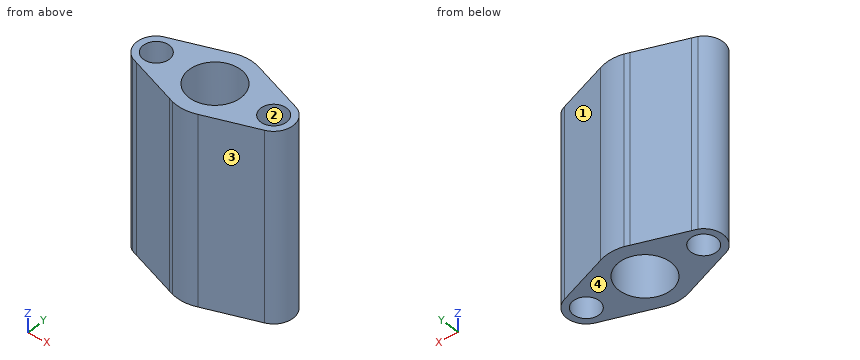
```python
from build123d import *

# Parameters (mm, degrees)
SKETCH5_R           = 10
SKETCH5_R_2         = 20
BOSS_EXTRUDE1_DEPTH = 147


with BuildPart() as part:
    # Sketch5 → Boss-Extrude1 (new body)
    with BuildSketch(Plane.XY):
        with BuildLine():
            Line((-95.000247062, 74.995110708), (-98.935518445, 73.594697295))
            ThreePointArc((-98.935518445, 73.594697295), (-106.987878642, 60.300702366), (-98.935518445, 47.006707437))
            Line((-98.935518445, 47.006707437), (-95.000247062, 45.606294025))
            Line((-95.000247062, 45.606294025), (-58.799859117, 32.723952789))
            Line((-58.799859117, 32.723952789), (-55.25219854, 31.46147532))
            ThreePointArc((-55.25219854, 31.46147532), (-45.821842976, 30.323371584), (-36.508384931, 32.190558084))
            Line((-36.508384931, 32.190558084), (3.010657963, 46.15804944))
            ThreePointArc((3.010657963, 46.15804944), (13.012121358, 60.300702366), (3.010657963, 74.443355293))
            Line((3.010657963, 74.443355293), (-36.508384931, 88.410846649))
            ThreePointArc((-36.508384931, 88.410846649), (-45.821842976, 90.278033149), (-55.25219854, 89.139929413))
            Line((-55.25219854, 89.139929413), (-58.799859117, 87.877451944))
            Line((-58.799859117, 87.877451944), (-95.000247062, 74.995110708))
        make_face()
        with Locations((-91.987878642, 60.300702366)):
            Circle(SKETCH5_R, mode=Mode.SUBTRACT)
        with Locations((-46.987878642, 60.300702366)):
            Circle(SKETCH5_R_2, mode=Mode.SUBTRACT)
        with Locations((-1.987878642, 60.300702366)):
            Circle(SKETCH5_R, mode=Mode.SUBTRACT)
    extrude(amount=-BOSS_EXTRUDE1_DEPTH)


solid = part.part
```
Part model, mm, in its own coordinate system. Face numbers are marked on the shaded views. Round coordinates to 2 decimals unless told otherwise and drop trailing zeros. Write each loop counter-clockwise with the first axis right and the second up, starting at its lowest first coordinate (ties: lowest second). Pieces come first, ordered by that corner, then holes. Notation, with made-up numbers: M -3,41 L 39,41 A16 cw 39,61 Z; hole C 84.25,74 d2. An arc over 180 degrees is marked long. One line per question, with ' | ' between items.
(1) Probe line 1 along X through (y, z) = (52, -51.5); line 2 along X through (y, z) = (64, -94.5); line 3 along Y through (x, z) = (-95.5, -21.5). List the from-to ranges inside material, lowest first.
Answer key:
line 1: x = -104.48 to -97.56, -86.41 to -65.18, -28.79 to -7.56, 3.59 to 10.51 | line 2: x = -106.52 to -101.28, -82.7 to -66.64, -27.33 to -11.28, 7.3 to 12.55 | line 3: y = 45.78 to 50.94, 69.66 to 74.82
(2) Saw through at B-B on z = -130. Write the cut outline in (x, y).
Answer key:
outline: M -98.94,47.01 L -55.25,31.46 A30 ccw -36.51,32.19 L 3.01,46.16 A15 ccw 3.01,74.44 L -36.51,88.41 A30 ccw -55.25,89.14 L -98.94,73.59 A15 ccw Z; hole C -91.99,60.3 d20; hole C -46.99,60.3 d40; hole C -1.99,60.3 d20
(3) Saw through at A-A on x = -47. Write the cut outline in (y, z).
Answer key:
outline: M 30.3,-147 L 40.3,-147 L 40.3,0 L 30.3,0 Z; M 80.3,-147 L 90.3,-147 L 90.3,0 L 80.3,0 Z
(4) Two-plate mould, pull along Y, no slides. Class the marked faces 1, 2, 3 and 4: released by +Y, released by -Y, zero draft, split by the parting line, or undercut.
Answer key:
face 1: released by +Y | face 2: undercut | face 3: released by -Y | face 4: zero draft
(5) Pin check, flat tips, straight feed: pin 1 (5 mm diameter, centred on x = -12.5, z = -59, fed in from -Y); pin 2 (23 mm diameter, centred on x = -91.99, y = 60.3, fed in from -Z); pin 3 (12 mm diameter, centred on y = 72.5, z = -112.5, fed in from -X); pin 4 (12 mm diameter, centred on x = -1.99, y = 60.3, fed in from +Z). Stop position of each tip, or through.
Answer key:
pin 1: stops at y = 39.79 | pin 2: stops at z = -147 | pin 3: stops at x = -105.65 | pin 4: passes through
(6) Saw through at D-D on y = 43.5. Write the cut outline in (x, z).
Answer key:
outline: M -89.08,-147 L -57.84,-147 L -57.84,0 L -89.08,0 Z; M -36.14,-147 L -4.51,-147 L -4.51,0 L -36.14,0 Z
(7) Saw through at C-C on y = 62.5. Write the cut outline in (x, z), then the cut area to 3 significant figures.
Answer key:
outline: M -106.83,-147 L -101.74,-147 L -101.74,0 L -106.83,0 Z; M -82.23,-147 L -66.87,-147 L -66.87,0 L -82.23,0 Z; M -27.11,-147 L -11.74,-147 L -11.74,0 L -27.11,0 Z; M 7.77,-147 L 12.85,-147 L 12.85,0 L 7.77,0 Z | area: 6,010 mm^2
